For this review, use the dimensioned drawing (mm, ordinates from the lowest corner) and the shaded views. A direction names the side the tool comes from. Coordinates: 2 decimals unless noted, no trailing zeros. Loops run counter-clockwise (first coordinate to the right, second up) from the corner with the lowest first, then second, coordinate; pieces in that order, holes last. Notation, with made-up numbers: M 41.5,79 L 72.5,79 A8 ccw 72.5,89 Z; hole C 55,76.25 d6. An arc over 180 degrees is marked long. Use CSV: the item, a comma, the result in double quotes. Start each with the question number.
1. Draft analysis for pull direction X (two halves, no side actions). For the marked faces 1, 2, 3 and 4, state which applies: +X half, -X half, draft (parallel to the pull), parting line (faces both ways), or undercut.
2. Add section C-C, the plane z = 32. Write out the cut boundary in (x, y).
3. For L1, parallel to Z at x = 62, y = 4.5; L2, parallel to Z at x = 65.5, y = 2.25 (1 decimal); L3, parallel to Y at x = 37.5, z = 4, list the stretches that pass through material, from the lowest coordinate up.
4. Clearance check with flat-ended pins moving along their axes: P1, Ø2, axis at x = 70, y = 5, coming from the -Z side; P2, Ø1.1, axis at x = 5, y = 5.5, coming from the +Z side. State where each tip first meets the part, or that it passes through.
5. Tool access review of the marked faces 5 and 6: name each direction out of +Z, -Z, +X, -X, +Y, -Y from which nothing blocks a thin tool from reaching the whole face with its end or side.
6. Add section B-B, the plane y = 8. Write out the cut boundary in (x, z).
7. Add section A-A, the plane x = 37.5. Write out the cut boundary in (y, z).
8. Add section D-D, the plane x = 62. Write out the cut boundary in (y, z).
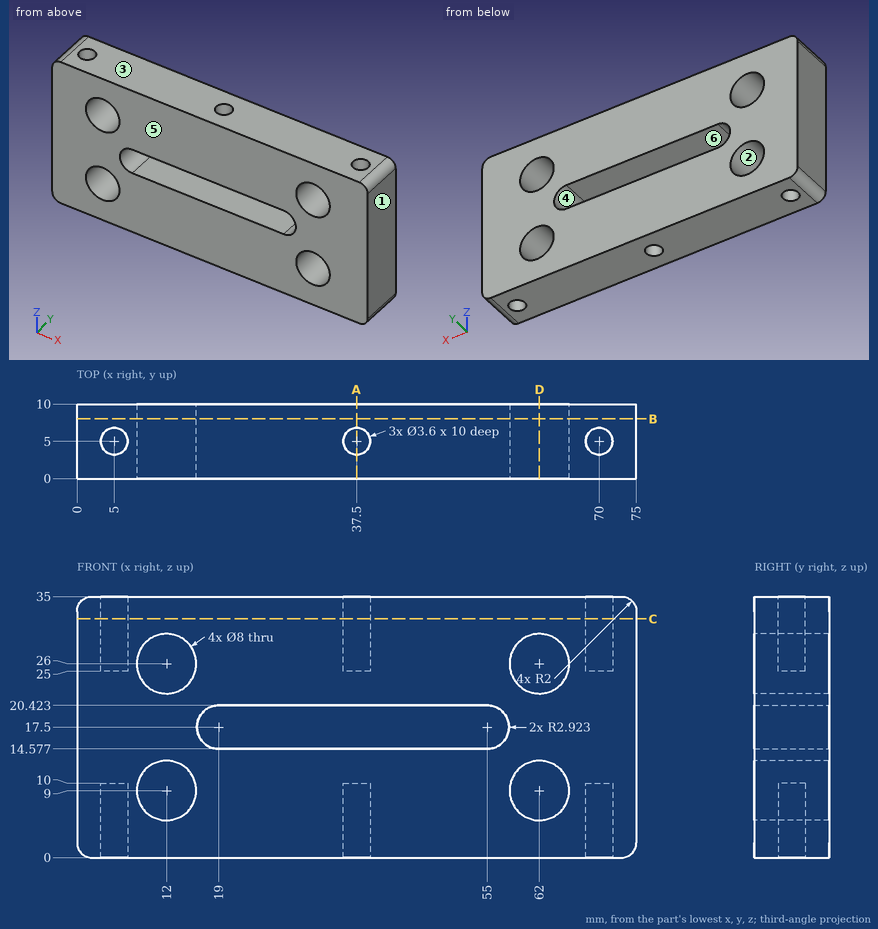
Computed:
1,face 1,"+X half"
1,face 2,"undercut"
1,face 3,"draft"
1,face 4,"undercut"
2,outline,"M 0,0 L 75,0 L 75,10 L 0,10 Z; hole C 5,5 d3.6; hole C 37.5,5 d3.6; hole C 70,5 d3.6"
3,L1,"z = 0 to 5, 13 to 22, 30 to 35"
3,L2,"z = 0 to 7.1, 10.9 to 24.1, 27.9 to 35"
3,L3,"y = 0 to 3.2, 6.8 to 10"
4,P1,"stops at z = 10"
4,P2,"stops at z = 25"
5,face 5,"+Z, -Z, +X, -X, -Y"
5,face 6,"+Y, -Y"
6,outline,"M 0,2 A2 ccw 2,0 L 73,0 A2 ccw 75,2 L 75,33 A2 ccw 73,35 L 2,35 A2 ccw 0,33 Z; hole C 12,9 d8; hole C 12,26 d8; hole M 19,14.58 L 55,14.58 A2.92 ccw 55,20.42 L 19,20.42 A2.92 ccw Z; hole C 62,9 d8; hole C 62,26 d8"
7,outline,"M 0,0 L 3.2,0 L 3.2,10 L 6.8,10 L 6.8,0 L 10,0 L 10,14.58 L 0,14.58 Z; M 0,20.42 L 10,20.42 L 10,35 L 6.8,35 L 6.8,25 L 3.2,25 L 3.2,35 L 0,35 Z"
8,outline,"M 0,0 L 10,0 L 10,5 L 0,5 Z; M 0,13 L 10,13 L 10,22 L 0,22 Z; M 0,30 L 10,30 L 10,35 L 0,35 Z"
